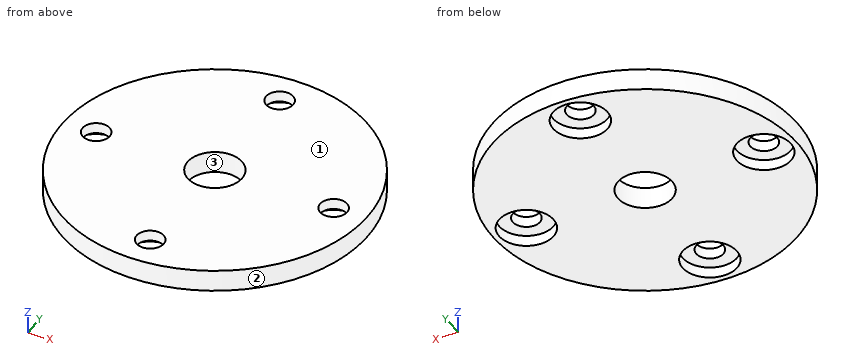
from build123d import *

# Parameters (mm, degrees)
SKETCH_R        = 14
SKETCH_R_2      = 1.25
PAD_DEPTH       = 2
SKETCH002_R     = 2.5
POCKET_DEPTH    = 9
SKETCH003_R     = 2.5
POCKET001_DEPTH = 1


with BuildPart() as part:
    # Sketch → Pad (new body)
    with BuildSketch(Plane.XY):
        Circle(SKETCH_R)
        with Locations((0, 11)):
            Circle(SKETCH_R_2, mode=Mode.SUBTRACT)
        with Locations((-11, 0)):
            Circle(SKETCH_R_2, mode=Mode.SUBTRACT)
        with Locations((0, -11)):
            Circle(SKETCH_R_2, mode=Mode.SUBTRACT)
        with Locations((11, 0)):
            Circle(SKETCH_R_2, mode=Mode.SUBTRACT)
    extrude(amount=PAD_DEPTH)

    # Sketch002 (on Face7 of Pad) → Pocket (cut)
    with BuildSketch(Plane.XY.offset(2)):
        Circle(SKETCH002_R)
    extrude(amount=-POCKET_DEPTH, mode=Mode.SUBTRACT)

    # Sketch003 (on Face2 of Pocket) → Pocket001 (cut)
    with BuildSketch(Plane(origin=(0, 0, 0), x_dir=(1, 0, 0), z_dir=(0, 0, -1))):
        with Locations((0, 11)):
            Circle(SKETCH003_R)
        with Locations((11, 0)):
            Circle(SKETCH003_R)
        with Locations((0, -11)):
            Circle(SKETCH003_R)
        with Locations((-11, 0)):
            Circle(SKETCH003_R)
    extrude(amount=-POCKET001_DEPTH, mode=Mode.SUBTRACT)


solid = part.part
Verification items for the finished model (mm, model axes). Face numbers are marked on the shaded views. Give positions to 0.01 mm unless a question says otherwise; leave off trailing zeros. Write each loop counter-clockwise with the first axis right and the second up, starting at its lowest first coordinate (ties: lowest second). Pieces come first, ordered by that corner, then holes. Notation, with made-up numbers: M 43.5,-17.5 L 48.5,-17.5 A14 cw 48.5,-9.5 Z; hole C 31.5,44.25 d1. An arc over 180 degrees is marked long. Put each result on its own line as item: value. Start each with the question number.
1. Section check A-A (x = 0). Record the cut outline in (y, z), and give its area (3 significant figures).
2. Draft check along X on the marked faces 1, 2 and 3. Enter one of: +X half, -X half, draft (parallel to the pull), parting line (faces both ways), or undercut.
3. Section check B-B (z = 1.5). Record the cut outline in (x, y).
4. Go/stop test with flat-tipped pins: pin 1 Ø3 at (x, y) = (0, 0) entering from -Z; pin 2 Ø1 at (x, y) = (-1.5, 3.5) entering from -Z; pin 3 Ø1.5 at (x, y) = (-1, 10) entering from -Z; pin 4 Ø1 at (y, z) = (11, 1.5) entering from -X. Record where each tip stops, or that it passes through.
5. Scan lines: line 1 along Y through (x, z) = (0, 1.2); line 2 along Y through (x, z) = (0, 0.25); line 3 along Z through (x, y) = (1, 10). Record each from-to range of solid material in increasing order. Write a range as [from, to].
6. Section check C-C (y = -0.75). Record the cut outline in (x, z), and give its area (3 significant figures).
7. Section check D-D (x = -11). Record the cut outline in (y, z), and give its area (3 significant figures).
Answer list:
1. outline: M -14,0 L -13.5,0 L -13.5,1 L -12.25,1 L -12.25,2 L -14,2 Z; M -9.75,1 L -8.5,1 L -8.5,0 L -2.5,0 L -2.5,2 L -9.75,2 Z; M 2.5,0 L 8.5,0 L 8.5,1 L 9.75,1 L 9.75,2 L 2.5,2 Z; M 12.25,1 L 13.5,1 L 13.5,0 L 14,0 L 14,2 L 12.25,2 Z
1. area: 31.0 mm2
2. face 1: draft
2. face 2: parting line
2. face 3: undercut
3. outline: C 0,0 d28; hole C -11,0 d2.5; hole C 0,0 d5; hole C 0,-11 d2.5; hole C 0,11 d2.5; hole C 11,0 d2.5
4. pin 1: through
4. pin 2: z = 0
4. pin 3: z = 1
4. pin 4: x = -9.26
5. line 1: [-14, -12.25], [-9.75, -2.5], [2.5, 9.75], [12.25, 14]
5. line 2: [-14, -13.5], [-8.5, -2.5], [2.5, 8.5], [13.5, 14]
5. line 3: [1, 2]
6. outline: M -13.98,0 L -13.38,0 L -13.38,1 L -12,1 L -12,2 L -13.98,2 Z; M -10,1 L -8.62,1 L -8.62,0 L -2.38,0 L -2.38,2 L -10,2 Z; M 2.38,0 L 8.62,0 L 8.62,1 L 10,1 L 10,2 L 2.38,2 Z; M 12,1 L 13.38,1 L 13.38,0 L 13.98,0 L 13.98,2 L 12,2 Z
6. area: 32.8 mm2
7. outline: M -8.66,0 L -2.5,0 L -2.5,1 L -1.25,1 L -1.25,2 L -8.66,2 Z; M 1.25,1 L 2.5,1 L 2.5,0 L 8.66,0 L 8.66,2 L 1.25,2 Z
7. area: 27.1 mm2
